from build123d import *

# Parameters (mm, degrees)
BOSS_EXTRUDE1_DEPTH = 2.29
CUT_EXTRUDE1_DEPTH  = 3
FILLET1_R           = 10
FILLET2_R           = 3


with BuildPart() as part:
    # Sketch1 → Boss-Extrude1 (new body)
    with BuildSketch(Plane(origin=(0, 0, 0), x_dir=(1, 0, 0), z_dir=(0, 1, 0))):
        with BuildLine():
            Line((1.5, 297.496218463), (1.5, 271.496218463))
            ThreePointArc((1.5, 271.496218463), (70.269464473, 262.249211634), (134.449071126, 235.872622221))
            Line((134.449071126, 235.872622221), (147.449071126, 258.389282719))
            ThreePointArc((147.449071126, 258.389282719), (76.998665918, 287.362933321), (1.5, 297.496218463))
        make_face()
    extrude(amount=BOSS_EXTRUDE1_DEPTH)

    # Sketch3 → Cut-Extrude1 (cut)
    with BuildSketch(Plane(origin=(0, 2.29, 0), x_dir=(1, 0, 0), z_dir=(0, 1, 0))):
        with BuildLine():
            Line((7.5, 271.396751344), (129.203185143, 238.786481168))
            Line((129.203185143, 238.786481168), (136.70589842, 251.781561758))
            ThreePointArc((136.70589842, 251.781561758), (74.15175015, 276.738099028), (7.5, 286.402177897))
            Line((7.5, 286.402177897), (7.5, 271.396751344))
        make_face()
    extrude(amount=-CUT_EXTRUDE1_DEPTH, mode=Mode.SUBTRACT)

    # Fillet1
    fillet1_edges = [part.edges().sort_by_distance(p)[0] for p in [
        (7.5, 1.145, -286.402177897),
        (136.70589842, 1.145, -251.781561758),
    ]]
    fillet(fillet1_edges, radius=FILLET1_R)

    # Fillet2
    fillet2_edges = [part.edges().sort_by_distance(p)[0] for p in [
        (7.5, 1.145, -271.396751344),
        (129.203185143, 1.145, -238.786481168),
    ]]
    fillet(fillet2_edges, radius=FILLET2_R)


solid = part.part
Part model, mm, in its own coordinate system. A direction names the side the tool comes from. Give positions to 0.01 mm unless a question says otherwise; leave off trailing zeros. Order: outer loops, then holes, each group sorted by start corner. A loop starts at its lowest first (then second) coordinate and runs counter-clockwise, first axis right, second up. Notation, with made-up numbers: (4.5, -32) -> (10.5, -32) arc R30 cw to (10.5, -10) -> close; hole circle Ø3 at (42.25, 69). An arc over 180 degrees is marked (long way). Use one line per item in the form item = value.
(1) Saw through at A-A (z = -278.5). Write the cut outline in (x, y).
Solution:
outline = (1.5, 0) -> (7.83, 0) -> (7.83, 2.29) -> (1.5, 2.29) -> close; (67.23, 0) -> (104.61, 0) -> (104.61, 2.29) -> (67.23, 2.29) -> close
(2) Tool access for faces 1 (the face through (6.63, 1.13, -272.35)), 2 (the face through (74, 0, -278)): list every direction of +Z, -Z, +X, -X, +Y, -Y with a clear straight run to the whole face (end or side of a thin tool).
Solution:
face_1 = +Z, +Y, -Y
face_2 = +Z, -Z, +X, -X, -Y
(3) Pull direction X, two halves, no side cores. Call faces 3 (the face through (10.573, 1.129, -283.159)), 4 (the face through (78.031, 1.129, -287.084)), 5 (the face through (132.422, 1.129, -250.509)), 6 (the face through (74, 2.29, -278)): +X half, -X half, draft (parallel to the pull), parting line (faces both ways), or undercut.
Solution:
face_3 = undercut
face_4 = +X half
face_5 = -X half
face_6 = draft
(4) Drill centre lines: line 1 (Z direction, x = 46.5, y = 2.2); line 2 (X direction, y = 0.85, z = -255.5); line 3 (X direction, y = 1.15, z = -244.5). Where is each one in solid material? Low to high. Write a range as from..to.
Solution:
line_1 = -293.84..-282.7
line_2 = 129.11..145.78
line_3 = 132.28..139.43
(5) Saw through at D-D (z = -245). Write the cut outline in (x, y).
Solution:
outline = (132.44, 0) -> (139.72, 0) -> (139.72, 2.29) -> (132.44, 2.29) -> close
(6) Saw through at B-B (y = 1.4). Write the cut outline in (x, z), then the cut area to 3 significant figures.
Solution:
outline = (1.5, -297.5) arc R297.5 ccw to (147.45, -258.39) -> (134.45, -235.87) arc R271.5 cw to (131.88, -237.32) arc R3 ccw to (130.74, -241.44) -> (131.48, -242.73) arc R10 cw to (127.26, -256.69) arc R286.5 cw to (18.13, -285.93) arc R10 cw to (7.5, -275.95) -> (7.5, -274.46) arc R3 ccw to (4.45, -271.46) arc R271.5 cw to (1.5, -271.5) -> close
area = 1,870 mm²
(7) Saw through at C-C (x = 52). Write the cut outline in (y, z).
Solution:
outline = (0, -292.92) -> (2.29, -292.92) -> (2.29, -281.74) -> (0, -281.74) -> close
